from build123d import *

# Parameters (mm, degrees)
F1_DEPTH = 63.5
F0_W     = 25.4
F0_H     = 19.05
F2_DEPTH = 25.4
F4_DEPTH = 12.7
F5_R     = 6.35


with BuildPart() as f1:
    # F0 (on Right) → F1 (new body, symmetric)
    with BuildSketch(Plane.YZ):
        Polygon((-41.275, 9.525), (-41.275, -9.525), (41.275, -9.525), (41.275, 9.525), (-22.225, 9.525), align=None)
    extrude(amount=F1_DEPTH, both=True)

    # F0 (on Right) → F2 (join, symmetric)
    with BuildSketch(Plane.YZ):
        with BuildLine():
            Line((-41.275, 27.0002), (-41.275, 9.525))
            Line((-41.275, 9.525), (-22.225, 9.525))
            Line((-22.225, 9.525), (-22.225, 27.0002))
            ThreePointArc((-22.225, 27.0002), (-30.6600167011, 49.7606132173), (-51.8906498109, 61.5269267575))
            add(Edge.make_bspline(
                [(-51.8906498109, 61.5269267575), (-53.6187990349, 61.680210909), (-55.3718909395, 61.8132821575), (-57.15, 61.9252)],
                knots=[108.5427292954, 108.5427292954, 108.5427292954, 108.5427292954, 111.5045361635, 111.5045361635, 111.5045361635, 111.5045361635], degree=3))
            Line((-57.15, 61.9252), (-60.325, 61.9252))
            Line((-60.325, 61.9252), (-60.325, 42.8752))
            Line((-60.325, 42.8752), (-57.15, 42.8752))
            ThreePointArc((-57.15, 42.8752), (-45.9246798487, 38.2255201513), (-41.275, 27.0002))
        make_face()
        with Locations((-73.025, 52.4002)):
            Rectangle(F0_W, F0_H)
    extrude(amount=F2_DEPTH, both=True)

    # F0 (on Right) → F3 (revolve)
    with BuildSketch(Plane.YZ):
        Polygon((-85.725, 38.1), (-85.725, 42.8752), (-85.725, 61.9252), (-85.725, 66.675), (-111.125, 66.675), (-111.125, 38.1), align=None)
    revolve(axis=Axis((0, -85.725, 52.3875), (0, 0, -1)))

    # F0 (on Right) → F4 (join, symmetric)
    with BuildSketch(Plane.YZ):
        with BuildLine():
            Line((-22.225, 9.525), (41.275, 9.525))
            add(Edge.make_bspline(
                [(41.275, 9.525), (41.275, 23.1452958025), (11.4416475843, 55.9094503662), (-51.8906498109, 61.5269267575)],
                knots=[0, 0, 0, 0, 108.5427292954, 108.5427292954, 108.5427292954, 108.5427292954], degree=3))
            ThreePointArc((-51.8906498109, 61.5269267575), (-30.6600167011, 49.7606132173), (-22.225, 27.0002))
            Line((-22.225, 27.0002), (-22.225, 9.525))
        make_face()
    extrude(amount=F4_DEPTH, both=True)

    # F5
    f5_edges = [f1.edges().sort_by_distance(p)[0] for p in [
        (-63.5, 41.275, 0),
        (-63.5, -41.275, 0),
        (63.5, 41.275, 0),
        (63.5, -41.275, 0),
    ]]
    fillet(f5_edges, radius=F5_R)


solid = f1.part
Design review of the part built by this model. Coordinates are the model's own, in mm. A direction names the side the tool comes from. Coordinates: 2 decimals unless noted, no trailing zeros. Order: outer loops, then holes, each group sorted by start corner. A loop starts at its lowest first (then second) coordinate and runs counter-clockwise, first axis right, second up. Notation, with made-up numbers: (86, 33) -> (128, 33) arc R22 cw to (128, 55) -> close; hole circle Ø6 at (15, 67.25). An arc over 180 degrees is marked (long way). Use one line per item in the form item = value. Start each with the question number.
(1) Insertion check: pin 1 (15 mm diameter, centred on x = -43, y = -11, fed in from +Z) (3 decimals); pin 2 (10 mm diameter, centred on x = -16, z = 21.5, fed in from +Y); pin 3 (1 mm diameter, centred on y = -42, z = 11.5, fed in from +X); pin 4 (2 mm diameter, centred on y = -54, z = 49.5, fed in from +X). Each pin has a flat end and moves straight along its axis. Give the tip position at first contact, or say it passes through.
(2) For faces 1 (the flat face through (-2, -60, 61.925)), 2 (the cylindrical face through (-18.96, -30.44, 49.5)), 3 (the flat face through (1, -41.275, 5)), list the 3-axis set-ups (+Z, -Z, +X, -X, +Y, -Y) from which the entire face can be reached by the end or side of a thin tool; tool diameter is ignored.
(3) The part is to be moulded in two halves that separate along Y. For faces 4 (the cylindrical face through (-61.59, 39.464, 0.133)), 5 (the cylindrical face through (0.4, -46, 38.3)), 6 (the flat face through (25.4, -47, 42)), say which applies: +Y half, -Y half, draft (parallel to the pull), parting line (faces both ways), or undercut.
(4) For probe 1 along Y at (x, z) = (20.5, 20) (3 decimals); probe 2 along Z at (x, y) = (45, 27) (3 decimals); probe 3 along Y at (x, z) = (-1, 62), list the stretches that pass through material, from the lowest coordinate up.
(5) Add section B-B on y = -82. State the section outline as (x, z) points (3 decimals).
(6) Add section A-A on x = -31. State the section outline as (y, z) points (3 decimals).
Answer block:
q1.pin_1 = 9.525
q1.pin_2 = 38.76
q1.pin_3 = through
q1.pin_4 = 25.4
q2.face_1 = +Z, +Y
q2.face_2 = +Z, -X, +Y
q2.face_3 = -Z, +X, -X, -Y
q3.face_4 = +Y half
q3.face_5 = undercut
q3.face_6 = draft
q4.probe_1 = -41.275 to -22.225
q4.probe_2 = -9.525 to 9.525
q4.probe_3 = -111.11 to -60.34
q5.outline = (-25.4, 42.875) -> (-25.125, 42.875) -> (-25.125, 38.1) -> (25.125, 38.1) -> (25.125, 42.875) -> (25.4, 42.875) -> (25.4, 61.925) -> (25.125, 61.925) -> (25.125, 66.675) -> (-25.125, 66.675) -> (-25.125, 61.925) -> (-25.4, 61.925) -> close
q6.outline = (-41.275, -9.525) -> (41.275, -9.525) -> (41.275, 9.525) -> (-41.275, 9.525) -> close
